Geometry: final body of the model. Coordinates: model frame, mm. Face numbers are marked on the shaded views. A direction names the side the tool comes from. Give positions to 0.01 mm unless a question says otherwise; leave off trailing zeros. Write each loop counter-clockwise with the first axis right and the second up, starting at its lowest first coordinate (ties: lowest second). Pieces come first, ordered by that corner, then holes.
Q1. Cut plane B-B on x = 1. Return the cut outline in (y, z), plus the area to 3 significant figures.
Q2. Cut plane C-C on z = 1.6. Return the cut outline in (x, y), plus the area to 3 significant figures.
Q3. Cut plane D-D on y = 7. Return the cut outline in (x, z), plus the area to 3 significant figures.
Q4. Draft query along X for the marked faces 1, 2 and 3. Return one class per face: pulls with the +X half, pulls with the -X half, needs draft (parallel to the pull), parting line crosses it, or undercut.
Q5. Reachability of the marked faces 4, 5 and 6 from +Z, -Z, +X, -X, +Y, -Y: full face, straight path, thin tool, end or side. Return the list, or none.
Q6. Pin query (flat end, axial travel): pin 1 (2 mm diameter, centred on y = 6.5, z = -0.5, fed in from -X); pin 2 (2.5 mm diameter, centred on x = -0.5, z = 1, fed in from +Y); pin 3 (2 mm diameter, centred on x = -0.5, y = 6.5, fed in from +Z); pin 4 (2 mm diameter, centred on y = 6.5, z = 0.5, fed in from +X). Return the tip coordinate at first contact, or that it passes through.
Q7. Line query: L1, parallel to Y at x = -0.25, z = 1.6; L2, parallel to X at y = 6.75, z = -0.5. Output: solid intervals per line, ascending.
Q8. Cut plane A-A on z = -1.2. Return the cut outline in (x, y), plus the area to 3 significant figures.
```python
from build123d import *

# Parameters (mm, degrees)
SKETCH1_W           = 4.8
SKETCH1_H           = 4.8
BOSS_EXTRUDE1_DEPTH = 4.8
SKETCH2_W           = 2.8
SKETCH2_H           = 2.8
BOSS_EXTRUDE2_DEPTH = 4
FILLET1_R           = 1
FILLET2_R           = 0.25
FILLET3_R           = 0.25


with BuildPart() as part:
    # Sketch1 → Boss-Extrude1 (new body)
    with BuildSketch(Plane(origin=(0, 0, 0), x_dir=(1, 0, 0), z_dir=(0, 1, 0))):
        Rectangle(SKETCH1_W, SKETCH1_H)
    extrude(amount=BOSS_EXTRUDE1_DEPTH)

    # Sketch2 → Boss-Extrude2 (add)
    with BuildSketch(Plane(origin=(0, 4.8, 0), x_dir=(1, 0, 0), z_dir=(0, 1, 0))):
        Rectangle(SKETCH2_W, SKETCH2_H)
    extrude(amount=BOSS_EXTRUDE2_DEPTH)

    # Fillet1
    fillet1_edges = [part.edges().sort_by_distance(p)[0] for p in [
        (1.4, 8.8, 0),
        (0, 8.8, -1.4),
        (-1.4, 8.8, 0),
        (0, 8.8, 1.4),
    ]]
    fillet(fillet1_edges, radius=FILLET1_R)

    # Fillet2
    fillet2_edges = [part.edges().sort_by_distance(p)[0] for p in [
        (0, 0, 2.4),
        (-2.4, 0, 0),
        (0, 0, -2.4),
        (2.4, 0, 0),
    ]]
    fillet(fillet2_edges, radius=FILLET2_R)

    # Fillet3
    # the kernel refuses this fillet: 0.25 mm, written as the material it takes off along each edge
    with BuildSketch(Plane(origin=(-2.15, 0.25, 2.15), x_dir=(0, 0, 1), z_dir=(-1, 0, 0))) as fillet3_piece_1_section:
        Polygon((0, 0), (FILLET3_R, 0), (FILLET3_R, -FILLET3_R), (0, -FILLET3_R), align=None)
    fillet3_piece_1 = extrude(amount=FILLET3_R, mode=Mode.PRIVATE)
    fillet3_piece_1 = fillet3_piece_1 - Plane(origin=(-2.15, 0.25, 2.15), x_dir=(0, 0.7071067811865475, -0.7071067811865475), z_dir=(-1, 0, 0)) * Sphere(FILLET3_R, mode=Mode.PRIVATE)
    add(fillet3_piece_1, mode=Mode.SUBTRACT)
    with BuildSketch(Plane(origin=(-2.15, 0.25, -2.15), x_dir=(-1, 0, 0), z_dir=(0, 0, -1))) as fillet3_piece_2_section:
        Polygon((0, 0), (FILLET3_R, 0), (FILLET3_R, -FILLET3_R), (0, -FILLET3_R), align=None)
    fillet3_piece_2 = extrude(amount=FILLET3_R, mode=Mode.PRIVATE)
    fillet3_piece_2 = fillet3_piece_2 - Plane(origin=(-2.15, 0.25, -2.15), x_dir=(0.7071067811865475, 0.7071067811865475, 0), z_dir=(0, 0, -1)) * Sphere(FILLET3_R, mode=Mode.PRIVATE)
    add(fillet3_piece_2, mode=Mode.SUBTRACT)
    with BuildSketch(Plane(origin=(-2.4, 4.8, 3.025), x_dir=(0, -1, 0), z_dir=(0, 0, -1))) as fillet3_piece_3:
        with BuildLine():
            CenterArc((FILLET3_R, -FILLET3_R), FILLET3_R, 90, 90)
            Line((0, -FILLET3_R), (0, 0))
            Line((0, 0), (FILLET3_R, 0))
        make_face()
    extrude(amount=6.05, mode=Mode.SUBTRACT)
    with BuildSketch(Plane(origin=(-2.4, 0.25, 2.4), x_dir=(0, 0, -1), z_dir=(0, 1, 0)), Plane(origin=(-2.4, 0.25, -2.4), x_dir=(1, 0, 0), z_dir=(0, 1, 0))) as fillet3_piece_4:
        with BuildLine():
            CenterArc((FILLET3_R, -FILLET3_R), FILLET3_R, 90, 90)
            Line((0, -FILLET3_R), (0, 0))
            Line((0, 0), (FILLET3_R, 0))
        make_face()
    extrude(amount=5.175, mode=Mode.SUBTRACT)


solid = part.part
```
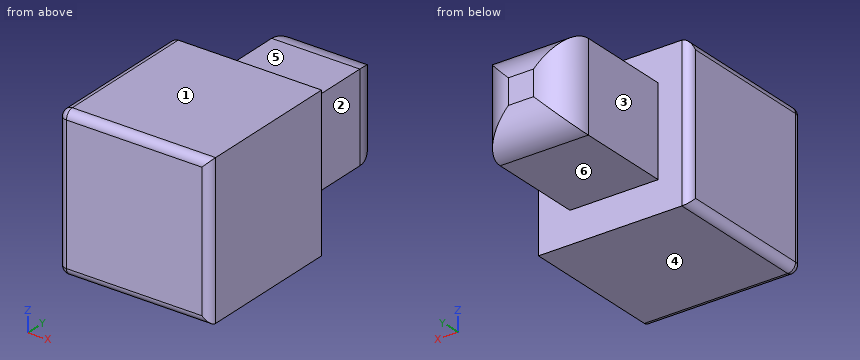
Data:
1. outline: (0, -2.15) arc R0.25 ccw to (0.25, -2.4) - (4.8, -2.4) - (4.8, -1.4) - (7.8, -1.4) arc R1 ccw to (8.6, -1) - (8.6, 1) arc R1 ccw to (7.8, 1.4) - (4.8, 1.4) - (4.8, 2.4) - (0.25, 2.4) arc R0.25 ccw to (0, 2.15) - close
1. area: 33.5 mm2
2. outline: (-2.4, 0.25) arc R0.25 ccw to (-2.15, 0) - (2.15, 0) arc R0.25 ccw to (2.4, 0.25) - (2.4, 4.8) - (-2.15, 4.8) arc R0.25 ccw to (-2.4, 4.55) - close
2. area: 23.0 mm2
3. outline: (-1.4, -1.4) - (1.4, -1.4) - (1.4, 1.4) - (-1.4, 1.4) - close
3. area: 7.84 mm2
4. face 1: needs draft
4. face 2: pulls with the +X half
4. face 3: pulls with the -X half
5. face 4: -Z, +X, -X, +Y, -Y
5. face 5: +Z, +X, -X, +Y
5. face 6: -Z, +X, -X, +Y
6. pin 1: stops at x = -1.4
6. pin 2: stops at y = 8.8
6. pin 3: stops at z = 1.4
6. pin 4: stops at x = 1.4
7. L1: y = 0 to 4.8
7. L2: x = -1.4 to 1.4
8. outline: (-2.4, 0.25) arc R0.25 ccw to (-2.15, 0) - (2.15, 0) arc R0.25 ccw to (2.4, 0.25) - (2.4, 4.8) - (1.4, 4.8) - (1.4, 7.8) arc R1 ccw to (1.2, 8.4) - (-1.2, 8.4) arc R1 ccw to (-1.4, 7.8) - (-1.4, 4.8) - (-2.15, 4.8) arc R0.25 ccw to (-2.4, 4.55) - close
8. area: 33.0 mm2
